Build history of the part. All positions in model axes, mm. Round coordinates to 2 decimals unless told otherwise and drop trailing zeros. Order: outer loops, then holes, each group sorted by start corner. A loop starts at its lowest first (then second) coordinate and runs counter-clockwise, first axis right, second up. Notation, with made-up numbers: (-32, -5) -> (9, -5) arc R12 cw to (9, 9) -> close; hole circle Ø6 at (10.5, 55.5). An arc over 180 degrees is marked (long way). Write item = value, one per line.
from build123d import *

# Parameters (mm, degrees)
BOSS_EXTRUDE1_DEPTH     = 10.16
SKETCH4_R               = 10.16
BOSS_EXTRUDE2_DEPTH     = 88.9
CUT_EXTRUDE1_DEPTH      = 160.369980112
CUT_EXTRUDE1_DEPTH_BACK = 160.369980112
SKETCH5_R               = 7.62


with BuildPart() as part:
    # Sketch1 → Boss-Extrude1 (new body)
    with BuildSketch(Plane(origin=(0, 0, 0), x_dir=(1, 0, 0), z_dir=(0, 1, 0))):
        with BuildLine():
            Line((0, 0), (27.899788868, 5.995845649))
            ThreePointArc((27.899788868, 5.995845649), (29.17117087, 6.158806163), (30.451880553, 6.106355894))
            Line((30.451880553, 6.106355894), (111.439136822, -4.081394546))
            ThreePointArc((111.439136822, -4.081394546), (122.553878894, -9.960729137), (127, -21.722364808))
            Line((127, -21.722364808), (127, -67.177635192))
            ThreePointArc((127, -67.177635192), (122.553878894, -78.939270863), (111.439136822, -84.818605454))
            Line((111.439136822, -84.818605454), (30.451880553, -95.006355894))
            ThreePointArc((30.451880553, -95.006355894), (29.17117087, -95.058806163), (27.899788868, -94.895845649))
            Line((27.899788868, -94.895845649), (0, -88.9))
            Line((0, -88.9), (0, 0))
        make_face()
    extrude(amount=BOSS_EXTRUDE1_DEPTH)

    # Sketch4 → Boss-Extrude2 (add)
    with BuildSketch(Plane.XY):
        with Locations((0, 5.08)):
            Circle(SKETCH4_R)
    extrude(amount=BOSS_EXTRUDE2_DEPTH)

    # Sketch5 → Cut-Extrude1 (cut, two sides: drawn at the far end of the back side and taken through both)
    with BuildSketch(Plane.XY.offset(-CUT_EXTRUDE1_DEPTH_BACK)):
        with Locations(Location((0, 5.08, 0), (0, 0, 41.810314896))):
            Circle(SKETCH5_R)
    extrude(amount=CUT_EXTRUDE1_DEPTH + CUT_EXTRUDE1_DEPTH_BACK, mode=Mode.SUBTRACT)


solid = part.part
Q1. Probe probe 1 along X at (y, z) = (5.08, 30); probe 2 along Y at (x, z) = (0, 33); probe 3 along X at (y, z) = (3.75, 31). List the from-to ranges inside material, lowest first.
Check values:
probe_1 = -10.16 to -7.62, 7.62 to 127
probe_2 = -5.08 to -2.54, 12.7 to 15.24
probe_3 = -10.07 to -7.5, 7.5 to 127
Q2. Flat gauge pins, fed straight in: pin 1 (3 mm diameter, centred on x = 84.5, z = 49, fed in from +Y); pin 2 (10 mm diameter, centred on y = -0.5, z = 77, fed in from -X); pin 3 (4 mm diameter, centred on x = 57.5, y = 6.5, fed in from -Z). Where does each tip first touch, or does it go through?
Check values:
pin_1 = 10.16
pin_2 = -10.14
pin_3 = -2.96
Q3. Cut at A-A, the plane x = 0. List the corners of the cut face in (y, z).
Check values:
outline = (-5.08, 0) -> (-2.54, 0) -> (-2.54, 88.9) -> (-5.08, 88.9) -> close; (12.7, 0) -> (15.24, 0) -> (15.24, 88.9) -> (12.7, 88.9) -> close
Q4. Mould opens along Y. For faces 1 (the face through (67, 10.16, 44)), 2 (the face through (67, 0, 44)), 3 (the face through (-1.416, -2.407, 43.804)), 4 (the face through (16.634, 5.009, -3.575)) say: released by +Y, released by -Y, zero draft, split by the parting line, or undercut.
Check values:
face_1 = released by +Y
face_2 = released by -Y
face_3 = undercut
face_4 = zero draft
Q5. Cut at D-D, the plane z = 16. List the corners of the cut face in (x, y), and give its area (3 significant figures).
Check values:
outline = (8.8, 0) -> (126.05, 0) -> (126.05, 10.16) -> (8.8, 10.16) arc R10.16 ccw (long way) to start; hole circle Ø15.24 at (0, 5.08)
area = 1,320 mm²
Q6. Cut at C-C, the plane z = 48. List the corners of the cut face in (x, y).
Check values:
outline = (8.8, 0) -> (127, 0) -> (127, 10.16) -> (8.8, 10.16) arc R10.16 ccw (long way) to start; hole circle Ø15.24 at (0, 5.08)
Q7. Cut at B-B, the plane y = 5.08. List the corners of the cut face in (x, z), and give its area (3 significant figures).
Check values:
outline = (-10.16, 0) -> (-7.62, 0) -> (-7.62, 88.9) -> (-10.16, 88.9) -> close; (7.62, -1.64) -> (27.9, -6) arc R7.62 ccw to (30.45, -6.11) -> (111.44, 4.08) arc R17.78 ccw to (127, 21.72) -> (127, 67.18) arc R17.78 ccw to (111.44, 84.82) -> (30.45, 95.01) arc R7.62 ccw to (27.9, 94.9) -> (7.62, 90.54) -> close
area = 10,900 mm²
